Geometry: final body of the model. Coordinates: model frame, mm. Face numbers are marked on the shaded views. A direction names the side the tool comes from. Give positions to 0.01 mm unless a question says otherwise; leave off trailing zeros. Write each loop counter-clockwise with the first axis right and the second up, starting at its lowest first coordinate (ties: lowest second). Pieces come first, ordered by that corner, then holes.
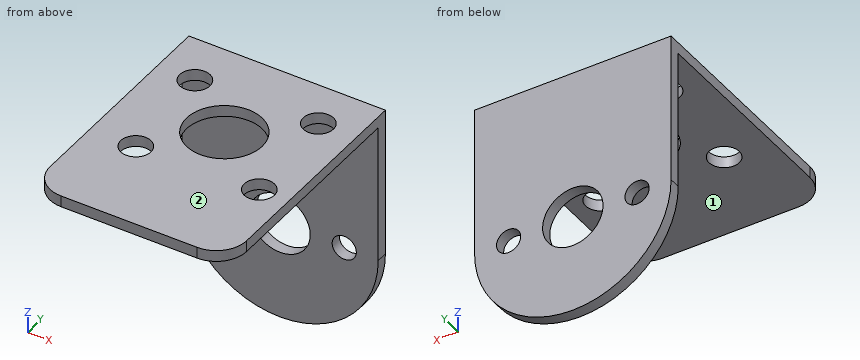
from build123d import *

# Parameters (mm, degrees)
SKETCH1_R           = 4
SKETCH1_R_2         = 1.6
BOSS_EXTRUDE1_DEPTH = 1.5
SKETCH2_R           = 5
SKETCH2_R_2         = 2
BOSS_EXTRUDE2_DEPTH = 1.5


with BuildPart() as part:
    # Sketch1 → Boss-Extrude1 (new body)
    with BuildSketch(Plane(origin=(0, 0, 0), x_dir=(1, 0, 0), z_dir=(0, 1, 0))):
        with BuildLine():
            Line((-13, -20), (-13, 0))
            ThreePointArc((-13, 0), (0, 13), (13, 0))
            Line((13, 0), (13, -20))
            Line((13, -20), (-13, -20))
        make_face()
        with Locations(Location((0, 0, 0), (0, 0, 270))):
            Circle(SKETCH1_R, mode=Mode.SUBTRACT)
        with Locations(Location((8.5, 0, 0), (0, 0, 270))):
            Circle(SKETCH1_R_2, mode=Mode.SUBTRACT)
        with Locations(Location((-8.5, 0, 0), (0, 0, 270))):
            Circle(SKETCH1_R_2, mode=Mode.SUBTRACT)
    extrude(amount=-BOSS_EXTRUDE1_DEPTH)

    # Sketch2 → Boss-Extrude2 (add)
    with BuildSketch(Plane.XY.offset(20)):
        with BuildLine():
            Line((13, -1.5), (13, -29))
            ThreePointArc((13, -29), (11.828427125, -31.828427125), (9, -33))
            Line((9, -33), (-9, -33))
            ThreePointArc((-9, -33), (-11.828427125, -31.828427125), (-13, -29))
            Line((-13, -29), (-13, -1.5))
            Line((-13, -1.5), (13, -1.5))
        make_face()
        with Locations((0, -13.122230355)):
            Circle(SKETCH2_R, mode=Mode.SUBTRACT)
        with Locations((8, -6.122230355)):
            Circle(SKETCH2_R_2, mode=Mode.SUBTRACT)
        with Locations((-8, -6.647631856)):
            Circle(SKETCH2_R_2, mode=Mode.SUBTRACT)
        with Locations((-6.942675301, -20.647631856)):
            Circle(SKETCH2_R_2, mode=Mode.SUBTRACT)
        with Locations((9.057324699, -20.122230355)):
            Circle(SKETCH2_R_2, mode=Mode.SUBTRACT)
    extrude(amount=-BOSS_EXTRUDE2_DEPTH)


solid = part.part
Q1. Pin query (flat end, axial travel): P1, Ø1.9, axis at x = -8.5, z = 0, coming from the -Y side; P2, Ø12, axis at x = 10, z = 11, coming from the +Y side; P3, Ø1.5, axis at x = 7, y = -8.5, coming from the -Z side; P4, Ø4, axis at x = 9.5, z = 15.5, coming from the -Y side. Return the tip coordinate at first contact, or that it passes through.
Filled sheet:
P1: passes through
P2: stops at y = 0
P3: stops at z = 18.5
P4: stops at y = -1.5
Q2. Ray query, line 1 along X through (y, z) = (-1.2, 0); line 2 along Y through (x, z) = (-8, 19.1); line 3 along Y through (x, z) = (-4.25, 5.5). Return the intervals inside material, ascending.
Filled sheet:
line 1: x = -13 to -10.1, -6.9 to -4, 4 to 6.9, 10.1 to 13
line 2: y = -33 to -22.35, -18.95 to -8.65, -4.65 to 0
line 3: y = -1.5 to 0
Q3. Section D-D on x = -8.5. Output: boundary loops of the cut face in (y, z), plus the area to 3 significant figures.
Filled sheet:
outline: (-33, 18.5) - (-21.9, 18.5) - (-21.9, 20) - (-33, 20) - close; (-19.39, 18.5) - (-8.58, 18.5) - (-8.58, 20) - (-19.39, 20) - close; (-4.71, 18.5) - (-1.5, 18.5) - (-1.5, 1.6) - (0, 1.6) - (0, 20) - (-4.71, 20) - close; (-1.5, -9.84) - (0, -9.84) - (0, -1.6) - (-1.5, -1.6) - close
area: 77.6 mm2
Q4. Section A-A on x = 0. Output: boundary loops of the cut face in (y, z).
Filled sheet:
outline: (-33, 18.5) - (-18.12, 18.5) - (-18.12, 20) - (-33, 20) - close; (-8.12, 18.5) - (-1.5, 18.5) - (-1.5, 4) - (0, 4) - (0, 20) - (-8.12, 20) - close; (-1.5, -13) - (0, -13) - (0, -4) - (-1.5, -4) - close
Q5. Access query for the marked faces 1 and 2. Directions: +Z, -Z, +X, -X, +Y, -Y. A direction counts if a zero-diameter tool reaches every point of the face in a straight line with its end or side. Return the directions, or none.
Filled sheet:
face 1: -Z, +X, -X, -Y
face 2: +Z, +X, -X, +Y, -Y
Q6. Section C-C on z = 0.5. Output: boundary loops of the cut face in (x, y), plus the area to 3 significant figures.
Filled sheet:
outline: (-13, -1.5) - (-10.02, -1.5) - (-10.02, 0) - (-13, 0) - close; (-6.98, -1.5) - (-3.97, -1.5) - (-3.97, 0) - (-6.98, 0) - close; (3.97, -1.5) - (6.98, -1.5) - (6.98, 0) - (3.97, 0) - close; (10.02, -1.5) - (13, -1.5) - (13, 0) - (10.02, 0) - close
area: 18.0 mm2
Q7. Section B-B on y = -12. Output: boundary loops of the cut face in (x, z).
Filled sheet:
outline: (-13, 18.5) - (-4.87, 18.5) - (-4.87, 20) - (-13, 20) - close; (4.87, 18.5) - (13, 18.5) - (13, 20) - (4.87, 20) - close
